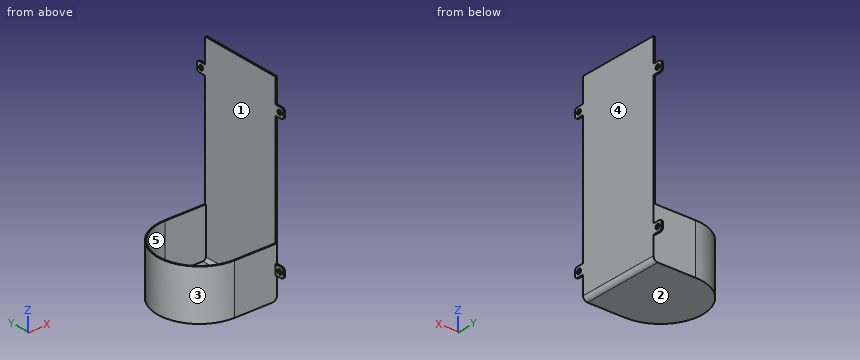
```python
from build123d import *

# Parameters (mm, degrees)
DODANIE_WYCI_GNI_CIE1_DEPTH = 1.5
SZKIC2_W                    = 1.5
SZKIC2_H                    = 86
DODANIE_WYCI_GNI_CIE2_DEPTH = 200
DODANIE_WYCI_GNI_CIE3_DEPTH = 50
ZAOKR_GLENIE1_R             = 3
ZAOKR_GLENIE2_R             = 4.5
DODANIE_WYCI_GNI_CIE4_DEPTH = 1.5
SZKIC6_R                    = 2.5
WYTNIJ_WYCI_GNI_CIE1_DEPTH  = 2.5


with BuildPart() as part:
    # Szkic1 → Dodanie-wyciągnięcie1 (new body)
    with BuildSketch(Plane.XY):
        with BuildLine():
            Line((-0.25, -43), (43.25, -43))
            Line((43.25, -43), (43.25, 43))
            Line((43.25, 43), (-0.25, 43))
            ThreePointArc((-0.25, 43), (-43.25, 0), (-0.25, -43))
        make_face()
    extrude(amount=DODANIE_WYCI_GNI_CIE1_DEPTH)

    # Szkic2 → Dodanie-wyciągnięcie2 (add)
    with BuildSketch(Plane.XY.offset(1.5)):
        with Locations((42.5, 0)):
            Rectangle(SZKIC2_W, SZKIC2_H)
    extrude(amount=DODANIE_WYCI_GNI_CIE2_DEPTH)

    # Szkic4 → Dodanie-wyciągnięcie3 (add)
    with BuildSketch(Plane.XY.offset(1.5)):
        with BuildLine():
            Line((-0.25, -43), (41.75, -43))
            Line((41.75, -43), (41.75, -42))
            Line((41.75, -42), (-0.25, -42))
            ThreePointArc((-0.25, -42), (-42.25, 0), (-0.25, 42))
            Line((-0.25, 42), (41.75, 42))
            Line((41.75, 42), (41.75, 43))
            Line((41.75, 43), (-0.25, 43))
            ThreePointArc((-0.25, 43), (-43.25, 0), (-0.25, -43))
        make_face()
    extrude(amount=DODANIE_WYCI_GNI_CIE3_DEPTH)

    # Zaokrąglenie1
    zaokr_glenie1_edges = [part.edges().sort_by_distance(p)[0] for p in [
        (41.75, 0, 1.5),
    ]]
    fillet(zaokr_glenie1_edges, radius=ZAOKR_GLENIE1_R)

    # Zaokrąglenie2
    zaokr_glenie2_edges = [part.edges().sort_by_distance(p)[0] for p in [
        (43.25, 0, 0),
    ]]
    fillet(zaokr_glenie2_edges, radius=ZAOKR_GLENIE2_R)

    # Szkic5 → Dodanie-wyciągnięcie4 (add)
    with BuildSketch(Plane.ZY.offset(-41.75)):
        with BuildLine():
            Line((166.5, 43), (176.5, 43))
            Line((176.5, 43), (176.5, 50))
            ThreePointArc((176.5, 50), (175.621320344, 52.121320344), (173.5, 53))
            Line((173.5, 53), (169.5, 53))
            ThreePointArc((169.5, 53), (167.378679656, 52.121320344), (166.5, 50))
            Line((166.5, 50), (166.5, 43))
        make_face()
        with BuildLine():
            Line((166.5, -50), (166.5, -43))
            Line((166.5, -43), (176.5, -43))
            Line((176.5, -43), (176.5, -50))
            ThreePointArc((176.5, -50), (175.621320344, -52.121320344), (173.5, -53))
            Line((173.5, -53), (169.5, -53))
            ThreePointArc((169.5, -53), (167.378679656, -52.121320344), (166.5, -50))
        make_face()
    dodanie_wyci_gni_cie4 = extrude(amount=-DODANIE_WYCI_GNI_CIE4_DEPTH)

    # Szkic6 → Wytnij-wyciągnięcie1 (cut, through all)
    with BuildSketch(Plane.ZY.offset(-41.75)):
        with Locations((171.5, 48)):
            Circle(SZKIC6_R)
        with Locations((171.5, -48)):
            Circle(SZKIC6_R)
    wytnij_wyci_gni_cie1 = extrude(amount=-WYTNIJ_WYCI_GNI_CIE1_DEPTH, mode=Mode.SUBTRACT)

    # Lustro1: Dodanie-wyciągnięcie4, Wytnij-wyciągnięcie1 across plane
    add(dodanie_wyci_gni_cie4.mirror(Plane.XY.offset(100)))
    add(wytnij_wyci_gni_cie1.mirror(Plane.XY.offset(100)), mode=Mode.SUBTRACT)


solid = part.part
```
Can you work these out from the model? Positions are in its coordinate system, mm. Face numbers are marked on the shaded views. A direction names the side the tool comes from. Coordinates: 2 decimals unless noted, no trailing zeros. Write each loop counter-clockwise with the first axis right and the second up, starting at its lowest first coordinate (ties: lowest second). Pieces come first, ordered by that corner, then holes. Notation, with made-up numbers: M -21,-33 L 38,-33 A22 ccw 38,-25 Z; hole C 46.5,22.5 d4. An arc over 180 degrees is marked long. Answer as CSV lines item,"result".
Item 1: I'm going to push flat-ended pins straight in: P1, Ø3, axis at y = -48, z = 28.5, coming from the +X side; P2, Ø1.6, axis at x = 42, z = 192, coming from the -Y side; P3, Ø2, axis at x = 19.5, y = 37.5, coming from the +Z side; P4, Ø0.8, axis at x = 42.5, y = 47.5, coming from the +Z side. Where does each tip first touch, or does it pass through?
Geometry results:
P1,"passes through"
P2,"stops at y = -43"
P3,"stops at z = 1.5"
P4,"stops at z = 176.5"
Item 2: Please list where these lines run through material, in increasing order: line 1 along Y through (x, z) = (42.15, 171.5); line 2 along Y through (x, z) = (29, 16.5); line 3 along Z through (x, y) = (3.5, -18.5).
Geometry results:
line 1,"y = -53 to -50.5, -45.5 to 45.5, 50.5 to 53"
line 2,"y = -43 to -42, 42 to 43"
line 3,"z = 0 to 1.5"
Item 3: We'd pull the mould along Y, two halves only. Please class the marked faces 3, 4 and 5: +Y half, -Y half, draft (parallel to the pull), parting line (faces both ways), or undercut.
Geometry results:
face 3,"parting line"
face 4,"draft"
face 5,"undercut"
Item 4: Imagine slicing it at D-D on y = 0. List the corners of the cut face in (x, z) for me, plus the area to 3 significant figures.
Geometry results:
outline,"M -43.25,0 L 38.75,0 A4.5 ccw 43.25,4.5 L 43.25,201.5 L 41.75,201.5 L 41.75,4.5 A3 cw 38.75,1.5 L -42.25,1.5 L -42.25,51.5 L -43.25,51.5 Z"
area,"477 mm2"
Item 5: Imagine slicing it at A-A on y = 48. List the corners of the cut face in (x, z) for me, plus the area to 3 significant figures.
Geometry results:
outline,"M 41.75,23.5 L 43.25,23.5 L 43.25,26 L 41.75,26 Z; M 41.75,31 L 43.25,31 L 43.25,33.5 L 41.75,33.5 Z; M 41.75,166.5 L 43.25,166.5 L 43.25,169 L 41.75,169 Z; M 41.75,174 L 43.25,174 L 43.25,176.5 L 41.75,176.5 Z"
area,"15.0 mm2"
Item 6: On a 3-axis mill with a long thin cutter (end or side, diameter ignored), from which of +Z, -Z, +X, -X, +Y, -Y can I reach the whole of each face in a straight line? I mean the marked faces 1 and 2. Say none if no direction works.
Geometry results:
face 1,"+Z"
face 2,"-Z, +X, -X, +Y, -Y"
Item 7: Imagine slicing it at C-C on x = 17.5. List the corners of the cut face in (y, z) for me, plus the area to 3 significant figures.
Geometry results:
outline,"M -43,0 L 43,0 L 43,51.5 L 42,51.5 L 42,1.5 L -42,1.5 L -42,51.5 L -43,51.5 Z"
area,"229 mm2"
Item 8: Imagine slicing it at B-B on z = 171.5. List the corners of the cut face in (x, y) for me.
Geometry results:
outline,"M 41.75,-53 L 43.25,-53 L 43.25,-50.5 L 41.75,-50.5 Z; M 41.75,-45.5 L 43.25,-45.5 L 43.25,45.5 L 41.75,45.5 Z; M 41.75,50.5 L 43.25,50.5 L 43.25,53 L 41.75,53 Z"
